Design review of the part built by this model. Coordinates are the model's own, in mm. Face numbers are marked on the shaded views. A direction names the side the tool comes from. Coordinates: 2 decimals unless noted, no trailing zeros. Order: outer loops, then holes, each group sorted by start corner. A loop starts at its lowest first (then second) coordinate and runs counter-clockwise, first axis right, second up. Notation, with made-up numbers: (60.5, 77.25) -> (96.5, 77.25) arc R31 cw to (96.5, 102.25) -> close; hole circle Ø6 at (-31.75, 14.5). An arc over 180 degrees is marked (long way). Write item = value, one per line.
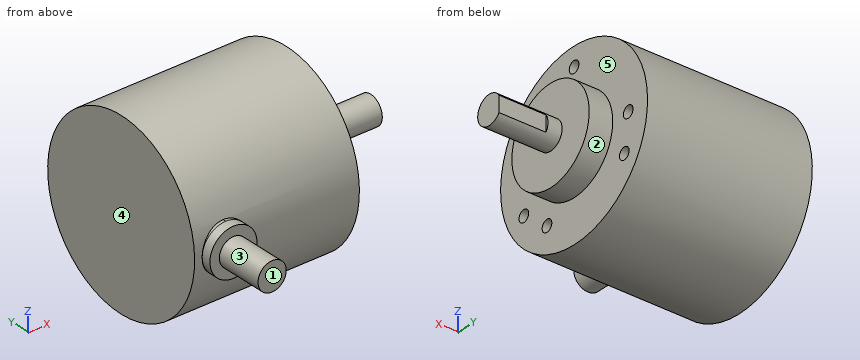
```python
from build123d import *
from build123d.topology import SkipClean

# Parameters (mm, degrees)
SKETCH1_R                            = 19
BOSS_EXTRUDE1_DEPTH                  = 35
SKETCH2_R                            = 10
BOSS_EXTRUDE2_DEPTH                  = 5
SKETCH3_R                            = 3
BOSS_EXTRUDE3_DEPTH                  = 13
SKETCH4_W                            = 10.869693714
SKETCH4_H                            = 3.318117029
CUT_EXTRUDE1_DEPTH                   = 10
SKETCH5_R                            = 5
BOSS_EXTRUDE4_DEPTH                  = 2
BOSS_EXTRUDE4_DIRECTION_2_REACH      = 69.926
BOSS_EXTRUDE4_DIRECTION_2_END_RADIUS = 19
SKETCH6_R                            = 3
BOSS_EXTRUDE5_DEPTH                  = 10
M3_TAPPED_HOLE1_AT_2_COUNT           = 2
M3_TAPPED_HOLE1_AT_2_PITCH           = 7.567650257
CIRPATTERN1_COUNT                    = 3


with BuildPart() as part:
    # Sketch1 → Boss-Extrude1 (new body)
    with BuildSketch(Plane(origin=(0, 0, 0), x_dir=(0, 0, -1), z_dir=(1, 0, 0))):
        Circle(SKETCH1_R)
    extrude(amount=BOSS_EXTRUDE1_DEPTH)

    # Sketch2 → Boss-Extrude2 (add)
    with BuildSketch(Plane(origin=(35, 0, 0), x_dir=(0, 0, -1), z_dir=(1, 0, 0))):
        Circle(SKETCH2_R)
    extrude(amount=BOSS_EXTRUDE2_DEPTH)

    # Sketch3 → Boss-Extrude3 (add)
    with BuildSketch(Plane(origin=(40, 0, 0), x_dir=(0, 0, -1), z_dir=(1, 0, 0))):
        with Locations(Location((0, 0, 0), (0, 0, 180))):
            Circle(SKETCH3_R)
    extrude(amount=BOSS_EXTRUDE3_DEPTH)

    # Sketch4 → Cut-Extrude1 (cut)
    with BuildSketch(Plane(origin=(53, 0, 0), x_dir=(0, 0, -1), z_dir=(1, 0, 0))):
        with Locations((-0.046103434, 4.159058514)):
            Rectangle(SKETCH4_W, SKETCH4_H)
    extrude(amount=-CUT_EXTRUDE1_DEPTH, mode=Mode.SUBTRACT)

    # Sketch5 → Boss-Extrude4 (add)
    with BuildSketch(Plane(origin=(0, -19, 0), x_dir=(-1, 0, 0), z_dir=(0, -1, 0))):
        with Locations(Location((-6.604465085, 0, 0), (0, 0, 270))):
            Circle(SKETCH5_R)
    extrude(amount=BOSS_EXTRUDE4_DEPTH)

    # Boss-Extrude4 direction 2: up to this cylinder (the profile starts outside it)
    with SkipClean():  # the faces are left unmerged after this step: merging them gives an invalid solid
        boss_extrude4_direction_2_end = Plane(origin=(6.604465, 0, 0), z_dir=(-1, 0, 0)) * Cylinder(BOSS_EXTRUDE4_DIRECTION_2_END_RADIUS, 178.852, mode=Mode.PRIVATE)
        # Sketch5 → Boss-Extrude4 direction 2 (add, up to the surface)
        with BuildSketch(Plane(origin=(0, -19, 0), x_dir=(-1, 0, 0), z_dir=(0, -1, 0)), mode=Mode.PRIVATE) as boss_extrude4_direction_2_sk1:
            with Locations(Location((-6.604465085, 0, 0), (0, 0, 270))):
                Circle(SKETCH5_R)
        boss_extrude4_direction_2_tool1 = extrude(boss_extrude4_direction_2_sk1.sketch, amount=-BOSS_EXTRUDE4_DIRECTION_2_REACH, mode=Mode.PRIVATE) - boss_extrude4_direction_2_end
        add(boss_extrude4_direction_2_tool1.solids().sort_by_distance((6.604465, -19, 0))[0])
        add(boss_extrude4_direction_2_tool1.solids().sort_by_distance((6.604465, -19, 0))[1])

    # Sketch6 → Boss-Extrude5 (add)
    with BuildSketch(Plane.XZ.offset(21)):
        with Locations(Location((6.604465085, 0, 0), (0, 0, 270))):
            Circle(SKETCH6_R)
    extrude(amount=BOSS_EXTRUDE5_DEPTH)

    # Sketch10 → M3 Tapped Hole1 (revolve, cut)
    with BuildSketch(Plane(origin=(35, 12.990381057, -7.5), x_dir=(0, 0, -1), z_dir=(0, 1, 0))):
        Polygon((0, 0), (0, 8.251075774), (1.25, 7.5), (1.25, 0), align=None)
    m3_tapped_hole1 = revolve(axis=Axis((41.35, 12.990381057, -7.5), (-1, 0, 0)), mode=Mode.SUBTRACT)

    # M3 Tapped Hole1 at 2: M3 Tapped Hole1 ×2
    with Locations(*[Vector(0, 0.13341247401263537, 0.9910605994477977) * (i * M3_TAPPED_HOLE1_AT_2_PITCH) for i in range(1, M3_TAPPED_HOLE1_AT_2_COUNT)]):
        add(m3_tapped_hole1, mode=Mode.SUBTRACT)

    # CirPattern1: M3 Tapped Hole1 ×3 about axis
    cirpattern1_axis = Axis((0, 0, 0), (1, 0, 0))
    for i in range(1, CIRPATTERN1_COUNT):
        add(m3_tapped_hole1.rotate(cirpattern1_axis, i * 360 / CIRPATTERN1_COUNT), mode=Mode.SUBTRACT)

    # CirPattern1 copy 1 sketch → CirPattern1 copy 1 (revolve, cut)
    with BuildSketch(Plane(origin=(35, -7, 12.124355653), x_dir=(0, 0.8660254037844387, 0.4999999999999998), z_dir=(0, -0.4999999999999998, 0.8660254037844387))):
        Polygon((0, 0), (0, 8.251075774), (1.25, 7.5), (1.25, 0), align=None)
    revolve(axis=Axis((41.35, -7, 12.124355653), (-1, 0, 0)), mode=Mode.SUBTRACT)

    # CirPattern1 copy 2 sketch → CirPattern1 copy 2 (revolve, cut)
    with BuildSketch(Plane(origin=(35, -7, -12.124355653), x_dir=(0, -0.8660254037844384, 0.5000000000000004), z_dir=(0, -0.5000000000000004, -0.8660254037844384))):
        Polygon((0, 0), (0, 8.251075774), (1.25, 7.5), (1.25, 0), align=None)
    revolve(axis=Axis((41.35, -7, -12.124355653), (-1, 0, 0)), mode=Mode.SUBTRACT)


solid = part.part
```
(1) For L1, parallel to Y at x = 31.25, z = -7.5; L2, parallel to X at y = 14.5, z = -3.5; L3, parallel to X at y = -0.5, z = -5, list the stretches that pass through material, from the lowest coordinate up.
Report:
L1 = -17.46 to -14.24, -11.74 to 11.74, 14.24 to 17.46
L2 = 0 to 35
L3 = 0 to 40
(2) We need section B-B (y = -20). Write out the cut boundary in (x, z), and give its area (3 significant figures).
Report:
outline = circle Ø10 at (6.6, 0)
area = 78.5 mm²
(3) Insertion check: pin 1 (4 mm diameter, centred on y = 5.5, z = -4.5, fed in from +X); pin 2 (12 mm diameter, centred on x = 27.5, z = -13, fed in from +Y); pin 3 (1.5 mm diameter, centred on y = -12.99, z = -7.5, fed in from +X). Each pin has a flat end and moves straight along its axis. Give the tip position at first contact, or say it passes through.
Report:
pin_1 = 40
pin_2 = 17.66
pin_3 = 27.2
(4) We need section A-A (z = 4). Write out the cut boundary in (x, y), and give its area (3 significant figures).
Report:
outline = (0, -18.57) -> (3.6, -18.57) -> (3.6, -21) -> (9.6, -21) -> (9.6, -18.57) -> (35, -18.57) -> (35, -9.17) -> (40, -9.17) -> (40, 9.17) -> (35, 9.17) -> (35, 18.57) -> (0, 18.57) -> close
area = 1,410 mm²
(5) For the marked faces 1 and 2, list the 3-axis set-ups (+Z, -Z, +X, -X, +Y, -Y) from which the entire face can be reached by the end or side of a thin tool; tool diameter is ignored.
Report:
face_1 = +Z, -Z, +X, -X, -Y
face_2 = +X
(6) We need section D-D (y = -11). Write out the cut boundary in (x, z), and give its area (3 significant figures).
Report:
outline = (0, -15.49) -> (35, -15.49) -> (35, 15.49) -> (0, 15.49) -> close
area = 1,080 mm²
(7) We need section C-C (z = 9). Write out the cut boundary in (x, y).
Report:
outline = (0, -16.73) -> (35, -16.73) -> (35, -4.36) -> (40, -4.36) -> (40, 4.36) -> (35, 4.36) -> (35, 16.73) -> (0, 16.73) -> close
(8) The part is to be moulded in two halves that separate along X. For the marked faces 3, 4 and 5, say which applies: released by +X, released by -X, zero draft, split by the parting line, or undercut.
Report:
face_3 = split by the parting line
face_4 = released by -X
face_5 = released by +X
